The listing builds one solid part. Answer for the finished solid, in the listing's coordinates (mm). A direction names the side the tool comes from. Round coordinates to 2 decimals unless told otherwise and drop trailing zeros. Loops run counter-clockwise (first coordinate to the right, second up) from the corner with the lowest first, then second, coordinate; pieces in that order, holes last. Notation, with made-up numbers: M 27,18.25 L 85,18.25 A26 ccw 85,48.25 Z; hole C 44,46.25 d6. An arc over 180 degrees is marked long. Put each result on its own line as item: value. Start each with the question number.
(1) Determine the mould class of faces 1 (the face through (-1, 39.706, 25)), 2 (the face through (-64.803, 0, 26)), 3 (the face through (76.151, -1, 25)) for opening direction X: released by +X, released by -X, zero draft, split by the parting line, or undercut.
(2) Which of the six approach directions +Z, -Z, +X, -X, +Y, -Y give full straight-line access (tool end or side, diameter ignored) to faces 4 (the face through (0, -34, 38.887)), 5 (the face through (-1, -27.617, 26)), 6 (the face through (-66, 1, 64.438))?
(3) Section B-B, the plane y = 25 is taken. Determine the outline of the cut face in (x, z), then the cut area to 3 significant figures.
(4) Straight lines are drawn through the part: line 1 (X direction, y = -22, z = 36); line 2 (Y direction, x = 48, z = 23.5); line 3 (X direction, y = 29, z = 41). For each, find the intervals that lie inside material, in ascending order.
(5) Section D-D, the plane z = 9.5 is taken. Determine the outline of the cut face in (x, y), then the cut area to 3 significant figures.
(6) A flat-ended cylindrical pin translates along its axis: P1, Ø13.5, axis at x = 15, y = 35.5, coming from the +Z side. Find the tip coordinate at first contact, or state that the pin passes through.
(7) Section C-C, the plane z = 45 is taken. Determine the outline of the cut face in (x, y), then the cut area to 3 significant figures.
(8) Section A-A, the plane x = 36.5 is taken. Determine the outline of the cut face in (y, z), then the cut area to 3 significant figures.
```python
from build123d import *

# Parameters (mm, degrees)
F0_W     = 152.3013710976
F0_H     = 79.4126093388
F1_DEPTH = 64.4375029951
F2_W     = 129.606127739
F2_H     = 55.234760046
F3_DEPTH = 64.4385029951
F7_W     = 76.3396583498
F7_H     = 25.5502108485
F4_DEPTH = 79.4136093388
F5_R     = 8.4271514965
F6_DEPTH = 152.3023710976


with BuildPart() as f1:
    # F0 (on Top) → F1 (new body)
    with BuildSketch(Plane.XY):
        Rectangle(F0_W, F0_H)
    extrude(amount=F1_DEPTH)

    # F2 (on face) → F3 (cut, through all)
    with BuildSketch(Plane.XY.offset(64.4375029951)):
        Rectangle(F2_W, F2_H)
    extrude(amount=-F3_DEPTH, mode=Mode.SUBTRACT)

    # F7 (on face) → F4 (cut, through all)
    with BuildSketch(Plane.XZ.offset(39.7063046694)):
        with Locations((0.1601595432, 51.6623975709)):
            Rectangle(F7_W, F7_H)
    extrude(amount=-F4_DEPTH, mode=Mode.SUBTRACT)

    # F5 (on face) → F6 (cut, through all)
    with BuildSketch(Plane.YZ.offset(76.1506855488)):
        with Locations((-0.2117939293, 34.9230654538)):
            Circle(F5_R)
    extrude(amount=-F6_DEPTH, mode=Mode.SUBTRACT)


solid = f1.part
```
Recorded:
1. face 1: zero draft
1. face 2: undercut
1. face 3: released by +X
2. face 4: +Z, +Y, -Y
2. face 5: +Z, -Z
2. face 6: +Z, +X, -X, +Y, -Y
3. outline: M -76.15,0 L -64.8,0 L -64.8,64.44 L -76.15,64.44 Z; M 64.8,0 L 76.15,0 L 76.15,64.44 L 64.8,64.44 Z
3. area: 1,460 mm²
4. line 1: x = -76.15 to -64.8, 64.8 to 76.15
4. line 2: y = -39.71 to -27.62, 27.62 to 39.71
4. line 3: x = -76.15 to -38.01, 38.33 to 76.15
5. outline: M -76.15,-39.71 L 76.15,-39.71 L 76.15,39.71 L -76.15,39.71 Z; hole M -64.8,-27.62 L 64.8,-27.62 L 64.8,27.62 L -64.8,27.62 Z
5. area: 4,940 mm²
6. P1: stops at z = 38.89
7. outline: M -76.15,-39.71 L -38.01,-39.71 L -38.01,-27.62 L -64.8,-27.62 L -64.8,27.62 L -38.01,27.62 L -38.01,39.71 L -76.15,39.71 Z; M 38.33,-39.71 L 76.15,-39.71 L 76.15,39.71 L 38.33,39.71 L 38.33,27.62 L 64.8,27.62 L 64.8,-27.62 L 38.33,-27.62 Z
7. area: 3,090 mm²
8. outline: M -39.71,0 L -27.62,0 L -27.62,38.89 L -39.71,38.89 Z; M 27.62,0 L 39.71,0 L 39.71,38.89 L 27.62,38.89 Z
8. area: 940 mm²
